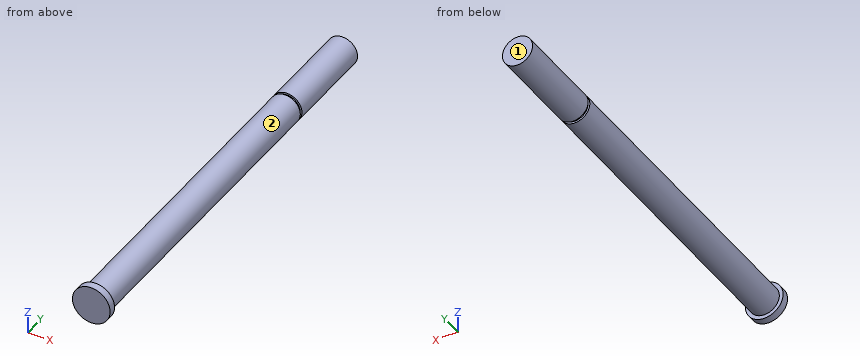
```python
from build123d import *

# Parameters (mm, degrees)
SKETCH1_R           = 4
BOSS_EXTRUDE1_DEPTH = 113
CUT_EXTRUDE1_START  = -0.75
SKETCH2_R           = 4
SKETCH2_R_2         = 3.5
CUT_EXTRUDE1_DEPTH  = 0.75
SKETCH3_R           = 5
BOSS_EXTRUDE2_DEPTH = 2


with BuildPart() as part:
    # Sketch1 → Boss-Extrude1 (new body)
    with BuildSketch(Plane(origin=(0, 0, 0), x_dir=(1, 0, 0), z_dir=(0, 1, 0))):
        with Locations(Location((0, 0, 0), (0, 0, 270))):
            Circle(SKETCH1_R)
    extrude(amount=BOSS_EXTRUDE1_DEPTH)

    # Sketch2 → Cut-Extrude1 (cut)
    with BuildSketch(Plane(origin=(0, 88, 0), x_dir=(1, 0, 0), z_dir=(0, 1, 0)).offset(CUT_EXTRUDE1_START)):
        with Locations(Location((0, 0, 0), (0, 0, 270))):
            Circle(SKETCH2_R)
        with Locations(Location((0, 0, 0), (0, 0, 270))):
            Circle(SKETCH2_R_2, mode=Mode.SUBTRACT)
    extrude(amount=CUT_EXTRUDE1_DEPTH, mode=Mode.SUBTRACT)

    # Sketch3 → Boss-Extrude2 (add)
    with BuildSketch(Plane(origin=(0, 0, 0), x_dir=(-1, 0, 0), z_dir=(0, -1, 0))):
        with Locations(Location((0, 0, 0), (0, 0, 90))):
            Circle(SKETCH3_R)
    extrude(amount=-BOSS_EXTRUDE2_DEPTH)


solid = part.part
```
Read the model definition and answer for the solid it produces. Units are mm, in the model's axes. Face numbers are marked on the shaded views. A direction names the side the tool comes from. Give positions to 0.01 mm unless a question says otherwise; leave off trailing zeros. Loops run counter-clockwise (first coordinate to the right, second up) from the corner with the lowest first, then second, coordinate; pieces in that order, holes last.
Item 1: The part is cut by section C-C (y = 38.5). Write down the section's boundary in (x, z), and give its area (3 significant figures).
Item 2: For the marked faces 1 and 2, determine the directions among +Z, -Z, +X, -X, +Y, -Y from which every point of the face is accessible in a straight line to the end or side of a thin tool.
Item 3: The part is cut by section B-B (x = -2.5). Write down the section's boundary in (y, z).
Item 4: The part is cut by section A-A (z = 0). Write down the section's boundary in (x, y), and give its area (3 significant figures).
Item 5: Find the intervals of material crossed by line 1 along X through (y, z) = (39, 0); line 2 along Y through (x, z) = (3.75, -2.25); line 3 along X through (y, z) = (49, -1.5), in increasing order.
Item 6: Each of these flat-tipped pins is pushed along its axis until it touches: pin 1 Ø6 at (x, y) = (-3.5, 84.5) entering from -Z; pin 2 Ø4 at (y, z) = (42, -2.5) entering from +X. Where does it stop, or does it pass through?
Taken from the geometry:
1. outline: circle Ø8 at (0, 0)
1. area: 50.3 mm2
2. face 1: +Z, -Z, +X, -X, +Y
2. face 2: +Y
3. outline: (0, -4.33) - (2, -4.33) - (2, -3.12) - (87.25, -3.12) - (87.25, -2.45) - (88, -2.45) - (88, -3.12) - (113, -3.12) - (113, 3.12) - (88, 3.12) - (88, 2.45) - (87.25, 2.45) - (87.25, 3.12) - (2, 3.12) - (2, 4.33) - (0, 4.33) - close
4. outline: (-5, 0) - (5, 0) - (5, 2) - (4, 2) - (4, 87.25) - (3.5, 87.25) - (3.5, 88) - (4, 88) - (4, 113) - (-4, 113) - (-4, 88) - (-3.5, 88) - (-3.5, 87.25) - (-4, 87.25) - (-4, 2) - (-5, 2) - close
4. area: 907 mm2
5. line 1: x = -4 to 4
5. line 2: y = 0 to 2
5. line 3: x = -3.71 to 3.71
6. pin 1: stops at z = -3.97
6. pin 2: stops at x = 3.97
